For this review, take the finished solid that the model builds, in its own axes (mm). Face numbers are marked on the shaded views. Give positions to 0.01 mm unless a question says otherwise; leave off trailing zeros. Order: outer loops, then holes, each group sorted by start corner. A loop starts at its lowest first (then second) coordinate and runs counter-clockwise, first axis right, second up.
Item 1: The part is to be moulded in two halves that separate along X. For the marked faces 1, 2, 3 and 4, say which applies: released by +X, released by -X, zero draft, split by the parting line, or undercut.
Item 2: Consider section A-A (z = 0). Give the boundary of the cut face in (x, y) (1 decimal).
Item 3: Consider section B-B (x = 0). Give the boundary of the cut face in (y, z) (1 decimal), plus the area to 3 significant figures.
Item 4: For P1, Ø8, axis at y = 6, z = -5, coming from the +X side; P2, Ø0.5, axis at x = 13, z = -20.5, coming from the +Y side (3 decimals); P3, Ø3, axis at y = 4, z = 15, coming from the +X side, all flat-tipped, find the tip position at first contact; note any pin that passes through.
Item 5: Consider section C-C (z = 13). Give the boundary of the cut face in (x, y) (3 decimals), plus the area to 3 significant figures.
Item 6: Consider section D-D (y = 14). Give the boundary of the cut face in (x, z) (1 decimal), plus the area to 3 significant figures.
Item 7: For probe 1 along X at (y, z) = (16.5, 0) (1 decimal); probe 2 along X at (y, z) = (2.5, 0); probe 3 along Y at (x, z) = (-7, -11), list the stretches that pass through material, from the lowest coordinate up.
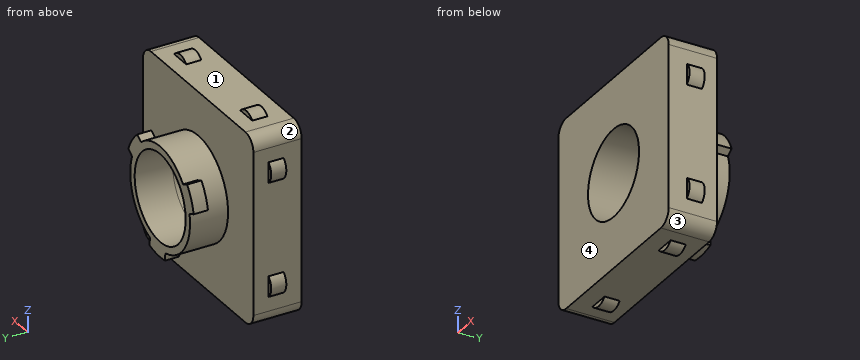
```python
from build123d import *

# Parameters (mm, degrees)
SKETCH1_W           = 39.8655
SKETCH1_H           = 39.8655
BOSS_EXTRUDE1_DEPTH = 10.16
SKETCH2_R           = 10.795
SKETCH2_R_2         = 9.2075
BOSS_EXTRUDE2_DEPTH = 8
BOSS_EXTRUDE3_START = -3
BOSS_EXTRUDE3_DEPTH = 3
CIRPATTERN1_COUNT   = 3
BOSS_EXTRUDE4_DEPTH = 6.35
CUT_EXTRUDE1_DEPTH  = 3.175
FILLET1_R           = 2.8575
SKETCH13_R          = 9.2075
CUT_EXTRUDE2_DEPTH  = 31.638540192
CIRPATTERN2_COUNT   = 4


with BuildPart() as part:
    # Sketch1 → Boss-Extrude1 (new body)
    with BuildSketch(Plane(origin=(0, 0, 0), x_dir=(1, 0, 0), z_dir=(0, 1, 0))):
        Rectangle(SKETCH1_W, SKETCH1_H)
    extrude(amount=BOSS_EXTRUDE1_DEPTH)

    # Sketch2 → Boss-Extrude2 (add)
    with BuildSketch(Plane(origin=(0, 10.16, 0), x_dir=(1, 0, 0), z_dir=(0, 1, 0))):
        with Locations(Location((0, 0, 0), (0, 0, 90))):
            Circle(SKETCH2_R)
        with Locations(Location((0, 0, 0), (0, 0, 270))):
            Circle(SKETCH2_R_2, mode=Mode.SUBTRACT)
    extrude(amount=BOSS_EXTRUDE2_DEPTH)

    # Sketch5 → Boss-Extrude3 (add)
    with BuildSketch(Plane(origin=(0, 18.16, 0), x_dir=(1, 0, 0), z_dir=(0, 1, 0)).offset(BOSS_EXTRUDE3_START)):
        with BuildLine():
            ThreePointArc((10.143998982, -3.692060354), (8.842746318, -6.19175763), (6.938853856, -8.269481977))
            Line((6.938853856, -8.269481977), (8.286221198, -9.212918747))
            ThreePointArc((8.286221198, -9.212918747), (10.150194049, -7.107242387), (11.491366324, -4.635497124))
            Line((11.491366324, -4.635497124), (10.143998982, -3.692060354))
        make_face()
    boss_extrude3 = extrude(amount=BOSS_EXTRUDE3_DEPTH)

    # CirPattern1: Boss-Extrude3 ×3 about axis
    cirpattern1_axis = Axis((0, 0, 0), (0, 1, 0))
    for i in range(1, CIRPATTERN1_COUNT):
        add(boss_extrude3.rotate(cirpattern1_axis, i * 360 / CIRPATTERN1_COUNT))

    # Sketch6 → Boss-Extrude4 (add)
    with BuildSketch(Plane(origin=(0, 10.16, 0), x_dir=(1, 0, 0), z_dir=(0, 1, 0))):
        with BuildLine():
            Line((-14.09175, 19.93275), (-9.77375, 19.93275))
            ThreePointArc((-9.77375, 19.93275), (-11.93275, 20.93275), (-14.09175, 19.93275))
        make_face()
        with BuildLine():
            Line((9.77375, 19.93275), (14.09175, 19.93275))
            ThreePointArc((14.09175, 19.93275), (11.93275, 20.93275), (9.77375, 19.93275))
        make_face()
    boss_extrude4 = extrude(amount=-BOSS_EXTRUDE4_DEPTH)

    # Sketch7 → Cut-Extrude1 (cut)
    with BuildSketch(Plane(origin=(0, 10.16, 0), x_dir=(1, 0, 0), z_dir=(0, 1, 0))):
        with BuildLine():
            Line((-9.77375, 19.93275), (-14.09175, 19.93275))
            ThreePointArc((-14.09175, 19.93275), (-11.93275, 20.93275), (-9.77375, 19.93275))
        make_face()
        with BuildLine():
            Line((9.77375, 19.93275), (14.09175, 19.93275))
            ThreePointArc((14.09175, 19.93275), (11.93275, 20.93275), (9.77375, 19.93275))
        make_face()
    cut_extrude1 = extrude(amount=-CUT_EXTRUDE1_DEPTH, mode=Mode.SUBTRACT)

    # Fillet1
    fillet1_edges = [part.edges().sort_by_distance(p)[0] for p in [
        (19.93275, 5.08, 19.93275),
        (-19.93275, 5.08, 19.93275),
        (-19.93275, 5.08, -19.93275),
        (19.93275, 5.08, -19.93275),
    ]]
    fillet(fillet1_edges, radius=FILLET1_R)

    # Sketch13 → Cut-Extrude2 (cut, through all)
    with BuildSketch(Plane(origin=(0, 10.16, 0), x_dir=(1, 0, 0), z_dir=(0, 1, 0))):
        with Locations(Location((0, 0, 0), (0, 0, 270))):
            Circle(SKETCH13_R)
    extrude(amount=-CUT_EXTRUDE2_DEPTH, mode=Mode.SUBTRACT)

    # CirPattern2: Boss-Extrude4, Cut-Extrude1 ×4 about axis
    cirpattern2_axis = Axis((0, 0, 0), (0, 1, 0))
    add([boss_extrude4.rotate(cirpattern2_axis, i * 360 / CIRPATTERN2_COUNT) for i in range(1, CIRPATTERN2_COUNT)])
    add([cut_extrude1.rotate(cirpattern2_axis, i * 360 / CIRPATTERN2_COUNT) for i in range(1, CIRPATTERN2_COUNT)], mode=Mode.SUBTRACT)


solid = part.part
```
Resolved:
1. face 1: undercut
1. face 2: released by -X
1. face 3: released by +X
1. face 4: zero draft
2. outline: (-19.9, 0) - (-9.2, 0) - (-9.2, 18.2) - (-10.8, 18.2) - (-10.8, 10.2) - (-19.9, 10.2) - close; (9.2, 0) - (19.9, 0) - (19.9, 10.2) - (10.8, 10.2) - (10.8, 18.2) - (9.2, 18.2) - close
3. outline: (0, -19.9) - (10.2, -19.9) - (10.2, -10.8) - (15.2, -10.8) - (15.2, -12.4) - (18.2, -12.4) - (18.2, -9.2) - (0, -9.2) - close; (0, 9.2) - (18.2, 9.2) - (18.2, 10.8) - (10.2, 10.8) - (10.2, 19.9) - (0, 19.9) - close
3. area: 248 mm2
4. P1: stops at x = 19.93
4. P2: stops at y = 6.985
4. P3: stops at x = 20.46
5. outline: (-20.724, 3.81) - (-19.933, 3.81) - (-19.933, 0) - (19.933, 0) - (19.933, 3.81) - (20.724, 3.81) - (20.724, 6.985) - (19.933, 6.985) - (19.933, 10.16) - (-19.933, 10.16) - (-19.933, 6.985) - (-20.724, 6.985) - close
5. area: 410 mm2
6. outline: circle Ø21.6 at (0, 0); hole circle Ø18.4 at (0, 0)
6. area: 99.8 mm2
7. probe 1: x = -10.8 to -9.2, 9.2 to 10.8
7. probe 2: x = -19.93 to -9.21, 9.21 to 19.93
7. probe 3: y = 0 to 10.16
